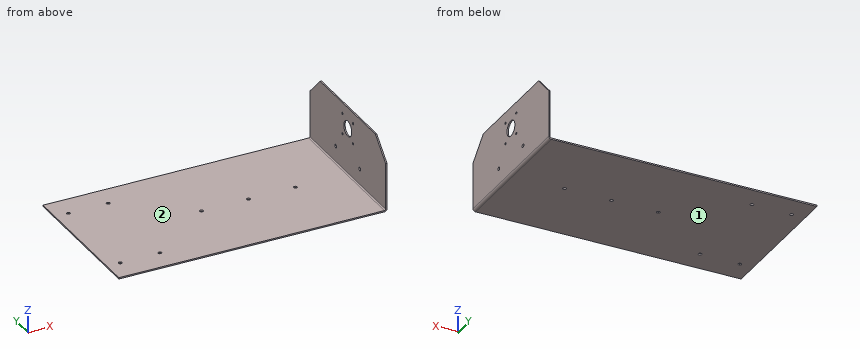
from build123d import *

# Parameters (mm, degrees)
SKETCH1_W            = 400
SKETCH1_H            = 220
BOSS_EXTRUDE1_DEPTH  = 3
SKETCH2_R            = 2.6
CUT_EXTRUDE1_DEPTH   = 90
SKETCH3_W            = 4
SKETCH3_H            = 220
BOSS_EXTRUDE2_DEPTH  = 90
SKETCH4_R            = 11.5
CUT_EXTRUDE2_DEPTH   = 90
SKETCH5_R            = 1.75
CUT_EXTRUDE3_DEPTH   = 90
SKETCH7_W            = 4
SKETCH7_H            = 220
BOSS_EXTRUDE3_DEPTH  = 10
CONVERT_SOLID2_START = -110
CONVERT_SOLID2_DEPTH = 220
CHAMFER1_SIZE        = 30
SKETCH6_R            = 2.6
CUT_EXTRUDE4_DEPTH   = 90


# Read off the part's stored shape, not the designer's step: Convert-Solid2
with BuildPart() as part:
    # Sketch1 → Boss-Extrude1 (new body)
    with BuildSketch(Plane.XY):
        Rectangle(SKETCH1_W, SKETCH1_H)
    extrude(amount=BOSS_EXTRUDE1_DEPTH)

    # Sketch2 → Cut-Extrude1 (cut)
    with BuildSketch(Plane(origin=(0, 0, 0), x_dir=(-1, 0, 0), z_dir=(0, 0, -1))):
        with Locations((-120, 0)):
            Circle(SKETCH2_R)
        with Locations((-50, 0)):
            Circle(SKETCH2_R)
        with Locations((20, 0)):
            Circle(SKETCH2_R)
        with Locations((120.81636457, -75.136060762)):
            Circle(SKETCH2_R)
        with Locations((120.81636457, 75.136060762)):
            Circle(SKETCH2_R)
        with Locations((180, 75.136060762)):
            Circle(SKETCH2_R)
        with Locations((180, -75.136060762)):
            Circle(SKETCH2_R)
    extrude(amount=-CUT_EXTRUDE1_DEPTH, mode=Mode.SUBTRACT)

    # Sketch3 → Boss-Extrude2 (add)
    with BuildSketch(Plane.XY.offset(3)):
        with Locations((198, 0)):
            Rectangle(SKETCH3_W, SKETCH3_H)
    extrude(amount=BOSS_EXTRUDE2_DEPTH)

    # Sketch4 → Cut-Extrude2 (cut)
    with BuildSketch(Plane(origin=(200, 0, 0), x_dir=(0, 0, -1), z_dir=(1, 0, 0))):
        with Locations(Location((-71, 0, 0), (0, 0, 90))):
            Circle(SKETCH4_R)
    extrude(amount=-CUT_EXTRUDE2_DEPTH, mode=Mode.SUBTRACT)

    # Sketch5 → Cut-Extrude3 (cut)
    with BuildSketch(Plane(origin=(200, 0, 0), x_dir=(0, 0, -1), z_dir=(1, 0, 0))):
        with Locations(Location((-55.5, 15.5, 0), (0, 0, 90))):
            Circle(SKETCH5_R)
        with Locations(Location((-55.5, -15.5, 0), (0, 0, 90))):
            Circle(SKETCH5_R)
        with Locations(Location((-86.5, -15.5, 0), (0, 0, 90))):
            Circle(SKETCH5_R)
        with Locations(Location((-86.5, 15.5, 0), (0, 0, 90))):
            Circle(SKETCH5_R)
    extrude(amount=-CUT_EXTRUDE3_DEPTH, mode=Mode.SUBTRACT)

    # Sketch7 → Boss-Extrude3 (add)
    with BuildSketch(Plane.XY.offset(93)):
        with Locations((198, 0)):
            Rectangle(SKETCH7_W, SKETCH7_H)
    extrude(amount=BOSS_EXTRUDE3_DEPTH)

    # Convert-Solid2 outline → Convert-Solid2 (cut)
    with BuildSketch(Plane(origin=(0, 0, 0), x_dir=(1, 0, 0), z_dir=(0, 1, 0)).offset(CONVERT_SOLID2_START)):
        with BuildLine():
            ThreePointArc((196.2, 0), (198.887005769, -1.112994231), (200, -3.8))
            Line((200, -3.8), (200, 0))
            Line((200, 0), (196.2, 0))
        make_face()
        with BuildLine():
            Line((196, -103), (198, -103))
            Line((198, -103), (198, -3.8))
            ThreePointArc((198, -3.8), (197.472792206, -2.527207794), (196.2, -2))
            Line((196.2, -2), (-200, -2))
            Line((-200, -2), (-200, -3))
            Line((-200, -3), (196, -3))
            Line((196, -3), (196, -103))
        make_face()
    extrude(amount=CONVERT_SOLID2_DEPTH, mode=Mode.SUBTRACT)

    # Chamfer1
    chamfer1_edges = [part.edges().sort_by_distance(p)[0] for p in [
        (199, -110, 103),
        (199, 110, 103),
    ]]
    chamfer(chamfer1_edges, length=CHAMFER1_SIZE)

    # Sketch6 → Cut-Extrude4 (cut)
    with BuildSketch(Plane(origin=(200, 0, 0), x_dir=(0, 0, -1), z_dir=(1, 0, 0))):
        with Locations(Location((-27, -35, 0), (0, 0, 90))):
            Circle(SKETCH6_R)
        with Locations(Location((-27, 35, 0), (0, 0, 90))):
            Circle(SKETCH6_R)
    extrude(amount=-CUT_EXTRUDE4_DEPTH, mode=Mode.SUBTRACT)


solid = part.part
For this review, take the finished solid that the model builds, in its own axes (mm). Face numbers are marked on the shaded views. A direction names the side the tool comes from. Round coordinates to 2 decimals unless told otherwise and drop trailing zeros. Order: outer loops, then holes, each group sorted by start corner. A loop starts at its lowest first (then second) coordinate and runs counter-clockwise, first axis right, second up. Notation, with made-up numbers: (-12.5, 0.25) -> (-8.5, 0.25) arc R28 cw to (-8.5, 19.25) -> close; hole circle Ø6 at (83, -23). An arc over 180 degrees is marked (long way). Write item = value, one per line. Start each with the question number.
1) Tool access review of the marked faces 1 and 2: name each direction out of +Z, -Z, +X, -X, +Y, -Y from which nothing blocks a thin tool from reaching the whole face with its end or side.
2) To check wall thickness, follow line 1 (Z direction, x = 198.85, y = -15.5); line 2 (Y direction, x = 198.75, z = 86.5); line 3 (Z direction, x = 143, y = -26). State the ranges of each line that lie inside material, in increasing order. Write a range as from..to.
3) Take a section at A-A on y = 87. State the section outline as (x, z) points, plus the area to 3 significant figures.
4) Take a section at B-B on z = 50. State the section outline as (x, y) points.
5) Insertion check: pin 1 (6 mm diameter, centred on y = -43.5, z = 41, fed in from -X); pin 2 (3 mm diameter, centred on x = 120, y = 0, fed in from +Z); pin 3 (7 mm diameter, centred on x = -20, y = 0, fed in from -Z); pin 4 (6 mm diameter, centred on x = -120.82, y = 75.14, fed in from +Z). Each pin has a flat end and moves straight along its axis. Give the tip position at first contact, or say it passes through.
6) Take a section at C-C on x = -85. State the section outline as (y, z) points.
Verdict:
q1.face_1 = -Z, +X, -X, +Y, -Y
q1.face_2 = +Z, -X, +Y, -Y
q2.line_1 = 1.08..53.75, 57.25..84.75, 88.25..103
q2.line_2 = -96.5..-17.25, -13.75..13.75, 17.25..96.5
q2.line_3 = 0..2
q3.outline = (-200, 0) -> (196.2, 0) arc R3.8 ccw to (200, 3.8) -> (200, 96) -> (198, 96) -> (198, 3.8) arc R1.8 cw to (196.2, 2) -> (-200, 2) -> close
q3.area = 986 mm2
q4.outline = (198, -110) -> (200, -110) -> (200, 110) -> (198, 110) -> close
q5.pin_1 = 198
q5.pin_2 = through
q5.pin_3 = 0
q5.pin_4 = 2
q6.outline = (-110, 0) -> (110, 0) -> (110, 2) -> (-110, 2) -> close
